```python
from build123d import *

# Parameters (mm, degrees)
F0_W     = 70
F0_H     = 55
F0_R     = 2
F0_R_2   = 1.55
F1_DEPTH = 1.5
F2_W     = 2
F2_H     = 51
F2_H_2   = 2
F2_W_2   = 20
F3_DEPTH = 3.5
F4_SIZE  = 3


with BuildPart() as f1:
    # F0 (on Top) → F1 (new body)
    with BuildSketch(Plane.XY):
        Rectangle(F0_W, F0_H)
        with Locations((-25, -17.5)):
            Circle(F0_R, mode=Mode.SUBTRACT)
        with Locations((31.45, -23.95)):
            Circle(F0_R_2, mode=Mode.SUBTRACT)
        with Locations((-25, 17.5)):
            Circle(F0_R, mode=Mode.SUBTRACT)
        with Locations((31.45, 23.95)):
            Circle(F0_R_2, mode=Mode.SUBTRACT)
    extrude(amount=-F1_DEPTH)

    # F2 (on face) → F3 (join)
    with BuildSketch(Plane.XY):
        with Locations((-14, 0)):
            Rectangle(F2_W, F2_H)
        Polygon((31.45, -25.5), (-13, -25.5), (-13, -27.5), (35, -27.5), (35, 27.5), (-13, 27.5), (-13, 25.5), (31.45, 25.5), (33, 25.5), (33, 23.95), (33, -23.95), (33, -25.5), align=None)
        with Locations((-14, -26.5)):
            Rectangle(F2_W, F2_H_2)
        with Locations((-25, -26.5)):
            Rectangle(F2_W_2, F2_H_2)
        with Locations((-14, 26.5)):
            Rectangle(F2_W, F2_H_2)
        with Locations((-25, 26.5)):
            Rectangle(F2_W_2, F2_H_2)
    extrude(amount=F3_DEPTH)

    # F4
    f4_edges = [f1.edges().sort_by_distance(p)[0] for p in [
        (-35, 26.5, 3.5),
        (-35, -26.5, 3.5),
    ]]
    chamfer(f4_edges, length=F4_SIZE)


solid = f1.part
```
Geometry check sheet. Reference: the model listing, model coordinates, mm. A direction names the side the tool comes from. Round coordinates to 2 decimals unless told otherwise and drop trailing zeros. Loops run counter-clockwise (first coordinate to the right, second up) from the corner with the lowest first, then second, coordinate; pieces in that order, holes last. Notation, with made-up numbers: (68.25, -10.75) -> (93.25, -10.75) arc R25 ccw to (93.25, 18.25) -> close; hole circle Ø3 at (70, -0.5). An arc over 180 degrees is marked (long way). Use a Markdown table: item, result.
(1) Sectioned sample at A-A (y = 17.5). Enter the section's corners in (x, z), then the cut area to 3 significant figures.
Calculated:
| item | result |
|---|---|
| outline | (-35, -1.5) -> (-27, -1.5) -> (-27, 0) -> (-35, 0) -> close; (-23, -1.5) -> (35, -1.5) -> (35, 3.5) -> (33, 3.5) -> (33, 0) -> (-13, 0) -> (-13, 3.5) -> (-15, 3.5) -> (-15, 0) -> (-23, 0) -> close |
| area | 113 mm² |
(2) Go/stop test with flat-tipped pins: P1, Ø1.8, axis at y = -7.5, z = 1.5, coming from the -X side; P2, Ø22, axis at x = -28, y = -3, coming from the +Z side. Record where each tip stops, or that it passes through.
Calculated:
| item | result |
|---|---|
| P1 | x = -15 |
| P2 | z = 0 |
(3) Sectioned sample at B-B (x = -10). Enter the section's corners in (y, z), then the cut area to 3 significant figures.
Calculated:
| item | result |
|---|---|
| outline | (-27.5, -1.5) -> (27.5, -1.5) -> (27.5, 3.5) -> (25.5, 3.5) -> (25.5, 0) -> (-25.5, 0) -> (-25.5, 3.5) -> (-27.5, 3.5) -> close |
| area | 96.5 mm² |
(4) Set-up check for faces 5 (the flat face through (-13, 0, 2)), 6 (the flat face through (-14, 0, 3.5)), 7 (the flat face through (-25, -25.5, 2)): record each of +Z, -Z, +X, -X, +Y, -Y from which the full face is reachable in a straight line by a thin tool's end or side.
Calculated:
| item | result |
|---|---|
| face 5 | +Z |
| face 6 | +Z, +X, -X, +Y, -Y |
| face 7 | +Z, -X |
(5) Mould release check, pull along Y, two halves, no side actions. Record for faces 1 (the flat face through (0, 27.5, 1)), 2 (the flat face through (-15, 0, 2)), 3 (the flat face through (-25, 0, 0)), 4 (the flat face through (-35, 0, -1)): released by +Y, released by -Y, zero draft, split by the parting line, or undercut.
Calculated:
| item | result |
|---|---|
| face 1 | released by +Y |
| face 2 | undercut |
| face 3 | undercut |
| face 4 | zero draft |
(6) Scan lines: probe 1 along Y at (x, z) = (-25, -0.5); probe 2 along X at (y, z) = (-14.5, 0.25); probe 3 along Y at (x, z) = (-18.5, 3.1). Record each from-to range of solid material in increasing order.
Calculated:
| item | result |
|---|---|
| probe 1 | -27.5 to -19.5, -15.5 to 15.5, 19.5 to 27.5 |
| probe 2 | -15 to -13, 33 to 35 |
| probe 3 | -27.5 to -25.5, 25.5 to 27.5 |
(7) Sectioned sample at C-C (y = -5). Enter the section's corners in (x, z).
Calculated:
| item | result |
|---|---|
| outline | (-35, -1.5) -> (35, -1.5) -> (35, 3.5) -> (33, 3.5) -> (33, 0) -> (-13, 0) -> (-13, 3.5) -> (-15, 3.5) -> (-15, 0) -> (-35, 0) -> close |
